Verification items for the finished model (mm, model axes). Coordinates: 2 decimals unless noted, no trailing zeros. Loops run counter-clockwise (first coordinate to the right, second up) from the corner with the lowest first, then second, coordinate; pieces in that order, holes last. Notation, with made-up numbers: (-22, 5.25) -> (34, 5.25) arc R25 ccw to (34, 17.25) -> close; hole circle Ø5 at (-36, -34.75). An arc over 180 degrees is marked (long way). Answer as a JSON object with one key per item and string values. Group by question number.
Q1. Release check for a two-part mould opening along Y. For faces 1 (the flat face through (0, 0, 2)), 2 (the flat face through (0, 2, 2)), 3 (the cylindrical face through (-3, 1, 0)) record: released by +Y, released by -Y, zero draft, split by the parting line, or undercut.
Q2. Cross-section at B-B on z = 0. Record the boundary of the cut face in (x, y), and give its area (3 significant figures).
Q3. Cross-section at D-D on z = -1. Record the boundary of the cut face in (x, y).
Q4. Cross-section at A-A on x = 0. Record the boundary of the cut face in (y, z).
Q5. Scan lines: L1, parallel to X at y = 0.65, z = 0; L2, parallel to X at y = 0.7, z = -1; L3, parallel to Z at x = -0.75, y = 0.9. Record each from-to range of solid material in increasing order.
Q6. Cross-section at C-C on y = 0.35. Record the boundary of the cut face in (x, z).
Q7. Gauge pin test, flat ends, axial feed: pin 1 Ø3 at (x, z) = (5.6, 0) entering from -Y; pin 2 Ø1 at (y, z) = (1.5, 3.5) entering from -X. Record the tip position at first contact, or that the pin passes through.
```python
from build123d import *

# Parameters (mm, degrees)
SKETCH_1_R      = 2.6
SKETCH_1_R_2    = 1.6
EXTRUDE_1_DEPTH = 2


with BuildPart() as part:
    # ｽｹｯﾁ1 → ﾎﾞｽ - 押し出し1 (new body)
    with BuildSketch(Plane(origin=(0, 0, 0), x_dir=(1, 0, 0), z_dir=(0, 1, 0))):
        with BuildLine():
            Line((-5.6, 5), (5.6, 5))
            ThreePointArc((5.6, 5), (10.6, 0), (5.6, -5))
            Line((5.6, -5), (-5.6, -5))
            ThreePointArc((-5.6, -5), (-10.6, 0), (-5.6, 5))
        make_face()
        with Locations(Location((-5.6, 0, 0), (0, 0, 270))):
            Circle(SKETCH_1_R, mode=Mode.SUBTRACT)
        with Locations(Location((5.6, 0, 0), (0, 0, 270))):
            Circle(SKETCH_1_R, mode=Mode.SUBTRACT)
        with Locations(Location((0, 0, 0), (0, 0, 270))):
            Circle(SKETCH_1_R_2, mode=Mode.SUBTRACT)
    extrude(amount=EXTRUDE_1_DEPTH)


solid = part.part
```
Computed values:
{
 "1": {"face 1": "released by -Y", "face 2": "released by +Y", "face 3": "zero draft"},
 "2": {"outline": "(-10.6, 0) -> (-8.2, 0) -> (-8.2, 2) -> (-10.6, 2) -> close; (-3, 0) -> (-1.6, 0) -> (-1.6, 2) -> (-3, 2) -> close; (1.6, 0) -> (3, 0) -> (3, 2) -> (1.6, 2) -> close; (8.2, 0) -> (10.6, 0) -> (10.6, 2) -> (8.2, 2) -> close", "area": "15.2 mm²"},
 "3": {"outline": "(-10.5, 0) -> (-8, 0) -> (-8, 2) -> (-10.5, 2) -> close; (-3.2, 0) -> (-1.25, 0) -> (-1.25, 2) -> (-3.2, 2) -> close; (1.25, 0) -> (3.2, 0) -> (3.2, 2) -> (1.25, 2) -> close; (8, 0) -> (10.5, 0) -> (10.5, 2) -> (8, 2) -> close"},
 "4": {"outline": "(0, -5) -> (2, -5) -> (2, -1.6) -> (0, -1.6) -> close; (0, 1.6) -> (2, 1.6) -> (2, 5) -> (0, 5) -> close"},
 "5": {"L1": "x = -10.6 to -8.2, -3 to -1.6, 1.6 to 3, 8.2 to 10.6", "L2": "x = -10.5 to -8, -3.2 to -1.25, 1.25 to 3.2, 8 to 10.5", "L3": "z = -5 to -1.41, 1.41 to 5"},
 "6": {"outline": "(-5.6, -5) -> (5.6, -5) arc R5 ccw to (5.6, 5) -> (-5.6, 5) arc R5 ccw to start; hole circle Ø5.2 at (-5.6, 0); hole circle Ø3.2 at (0, 0); hole circle Ø5.2 at (5.6, 0)"},
 "7": {"pin 1": "passes through", "pin 2": "stops at x = -9.6"}
}
